```python
from build123d import *

# Parameters (mm, degrees)
BOSS_EXTRUDE3_OUTLINE_R = 7.6
BOSS_EXTRUDE3_DEPTH     = 5
SKETCH2_R               = 1.6
CUT_EXTRUDE1_DEPTH      = 10
SKETCH3_R               = 1.6
CUT_EXTRUDE2_DEPTH      = 10
SKETCH4_R               = 1.5
CUT_EXTRUDE3_DEPTH      = 10
SKETCH5_R               = 3.25
CUT_EXTRUDE4_DEPTH      = 1.5
CUT_EXTRUDE5_DEPTH      = 10
FILLET1_R               = 2
FILL_PATTERN1_DEPTH     = 5
CUT_EXTRUDE6_DEPTH      = 10
FILLET2_R               = 2
FILL_PATTERN2_DEPTH     = 5


# Read off the part's stored shape, not the designer's step: Boss-Extrude3, Fill Pattern1, Fill Pattern2
with BuildPart() as part:
    # Boss-Extrude3 outline → Boss-Extrude3 (new body)
    with BuildSketch(Plane(origin=(0, 0, 0), x_dir=(1, 0, 0), z_dir=(0, 1, 0))):
        with BuildLine():
            ThreePointArc((0, 42.5), (-42.5, 0), (0, -42.5))
            add(Edge.make_bspline(
                [(0, -42.5), (50, -42.5), (76.766110149, 8.415768242), (141.161165235, -8.838834765)],
                knots=[0, 0, 0, 0, 1, 1, 1, 1], degree=3))
            ThreePointArc((141.161165235, -8.838834765), (158.838834765, -8.838834765), (158.838834765, 8.838834765))
            add(Edge.make_bspline(
                [(0, 42.5), (53.483495706, 42.5), (123.483495706, 44.194173824), (158.838834765, 8.838834765)],
                knots=[0, 0, 0, 0, 1, 1, 1, 1], degree=3))
        make_face()
        with Locations((150, 0)):
            Circle(BOSS_EXTRUDE3_OUTLINE_R, mode=Mode.SUBTRACT)
    extrude(amount=BOSS_EXTRUDE3_DEPTH)

    # Sketch2 → Cut-Extrude1 (cut)
    with BuildSketch(Plane(origin=(0, 5, 0), x_dir=(1, 0, 0), z_dir=(0, 1, 0))):
        with Locations(Location((0, 35, 0), (0, 0, 270))):
            Circle(SKETCH2_R)
        with Locations(Location((0, 11, 0), (0, 0, 270))):
            Circle(SKETCH2_R)
        with Locations(Location((9.526279442, 5.5, 0), (0, 0, 270))):
            Circle(SKETCH2_R)
        with Locations(Location((9.526279442, -5.5, 0), (0, 0, 270))):
            Circle(SKETCH2_R)
        with Locations(Location((0, -11, 0), (0, 0, 270))):
            Circle(SKETCH2_R)
        with Locations(Location((-9.526279442, -5.5, 0), (0, 0, 270))):
            Circle(SKETCH2_R)
        with Locations(Location((-9.526279442, 5.5, 0), (0, 0, 270))):
            Circle(SKETCH2_R)
        with Locations(Location((-20.57248383, 28.315594803, 0), (0, 0, 270))):
            Circle(SKETCH2_R)
        with Locations(Location((-33.28697807, 10.815594803, 0), (0, 0, 270))):
            Circle(SKETCH2_R)
        with Locations(Location((-33.28697807, -10.815594803, 0), (0, 0, 270))):
            Circle(SKETCH2_R)
        with Locations(Location((-20.57248383, -28.315594803, 0), (0, 0, 270))):
            Circle(SKETCH2_R)
        with Locations(Location((0, -35, 0), (0, 0, 270))):
            Circle(SKETCH2_R)
    extrude(amount=-CUT_EXTRUDE1_DEPTH, mode=Mode.SUBTRACT)

    # Sketch3 → Cut-Extrude2 (cut)
    with BuildSketch(Plane(origin=(0, 5, 0), x_dir=(1, 0, 0), z_dir=(0, 1, 0))):
        with Locations(Location((29.822508304, 35, 0), (0, 0, 270))):
            Circle(SKETCH3_R)
        with Locations(Location((57.312909887, 35, 0), (0, 0, 270))):
            Circle(SKETCH3_R)
    extrude(amount=-CUT_EXTRUDE2_DEPTH, mode=Mode.SUBTRACT)

    # Sketch4 → Cut-Extrude3 (cut)
    with BuildSketch(Plane(origin=(0, 5, 0), x_dir=(1, 0, 0), z_dir=(0, 1, 0))):
        with Locations(Location((22.392043347, -28.36049342, 0), (0, 0, 270))):
            Circle(SKETCH4_R)
    extrude(amount=-CUT_EXTRUDE3_DEPTH, mode=Mode.SUBTRACT)

    # Sketch5 → Cut-Extrude4 (cut)
    with BuildSketch(Plane.XZ):
        with Locations(Location((0, 11, 0), (0, 0, 270))):
            Circle(SKETCH5_R)
        with Locations(Location((9.526279442, 5.5, 0), (0, 0, 270))):
            Circle(SKETCH5_R)
        with Locations(Location((9.526279442, -5.5, 0), (0, 0, 270))):
            Circle(SKETCH5_R)
        with Locations(Location((0, -11, 0), (0, 0, 270))):
            Circle(SKETCH5_R)
        with Locations(Location((-9.526279442, -5.5, 0), (0, 0, 270))):
            Circle(SKETCH5_R)
        with Locations(Location((-9.526279442, 5.5, 0), (0, 0, 270))):
            Circle(SKETCH5_R)
    extrude(amount=-CUT_EXTRUDE4_DEPTH, mode=Mode.SUBTRACT)

    # Sketch6 → Cut-Extrude5 (cut)
    with BuildSketch(Plane(origin=(0, 5, 0), x_dir=(1, 0, 0), z_dir=(0, 1, 0))):
        Polygon((43, 27.773502692), (23, 27.773502692), (33, 10.452994616), align=None)
    extrude(amount=-CUT_EXTRUDE5_DEPTH, mode=Mode.SUBTRACT)

    # Fillet1
    fillet1_edges = [part.edges().sort_by_distance(p)[0] for p in [
        (43, 2.5, -27.773502692),
        (33, 2.5, -10.452994616),
        (23, 2.5, -27.773502692),
    ]]
    fillet(fillet1_edges, radius=FILLET1_R)

    # Fill Pattern1 outline → Fill Pattern1 (cut)
    with BuildSketch(Plane(origin=(0, 0, 0), x_dir=(1, 0, 0), z_dir=(0, 1, 0))):
        with BuildLine():
            ThreePointArc((41.464101615, 1.792740578), (39.732050808, 0.792740578), (39.732050808, -1.207259422))
            Line((39.732050808, -1.207259422), (46.267949192, -12.527767497))
            ThreePointArc((46.267949192, -12.527767497), (48, -13.527767497), (49.732050808, -12.527767497))
            Line((49.732050808, -12.527767497), (56.267949192, -1.207259422))
            ThreePointArc((56.267949192, -1.207259422), (56.267949192, 0.792740578), (54.535898385, 1.792740578))
            Line((54.535898385, 1.792740578), (41.464101615, 1.792740578))
        make_face()
        with BuildLine():
            ThreePointArc((101.267949192, 24.773502692), (101.267949192, 26.773502692), (99.535898385, 27.773502692))
            Line((99.535898385, 27.773502692), (86.464101615, 27.773502692))
            ThreePointArc((86.464101615, 27.773502692), (84.732050808, 26.773502692), (84.732050808, 24.773502692))
            Line((84.732050808, 24.773502692), (91.267949192, 13.452994616))
            ThreePointArc((91.267949192, 13.452994616), (93, 12.452994616), (94.732050808, 13.452994616))
            Line((94.732050808, 13.452994616), (101.267949192, 24.773502692))
        make_face()
        with BuildLine():
            ThreePointArc((71.267949192, 24.773502692), (71.267949192, 26.773502692), (69.535898385, 27.773502692))
            Line((69.535898385, 27.773502692), (56.464101615, 27.773502692))
            ThreePointArc((56.464101615, 27.773502692), (54.732050808, 26.773502692), (54.732050808, 24.773502692))
            Line((54.732050808, 24.773502692), (61.267949192, 13.452994616))
            ThreePointArc((61.267949192, 13.452994616), (63, 12.452994616), (64.732050808, 13.452994616))
            Line((64.732050808, 13.452994616), (71.267949192, 24.773502692))
        make_face()
    extrude(amount=FILL_PATTERN1_DEPTH, mode=Mode.SUBTRACT)

    # Sketch8 → Cut-Extrude6 (cut)
    with BuildSketch(Plane(origin=(0, 5, 0), x_dir=(1, 0, 0), z_dir=(0, 1, 0))):
        Polygon((58, 7.56624327), (48, 24.886751346), (38, 7.56624327), align=None)
    extrude(amount=-CUT_EXTRUDE6_DEPTH, mode=Mode.SUBTRACT)

    # Fillet2
    fillet2_edges = [part.edges().sort_by_distance(p)[0] for p in [
        (58, 2.5, -7.56624327),
        (38, 2.5, -7.56624327),
        (48, 2.5, -24.886751346),
    ]]
    fillet(fillet2_edges, radius=FILLET2_R)

    # Fill Pattern2 outline → Fill Pattern2 (cut)
    with BuildSketch(Plane(origin=(0, 0, 0), x_dir=(1, 0, 0), z_dir=(0, 1, 0))):
        with BuildLine():
            ThreePointArc((69.732050808, 10.56624327), (69.732050808, 8.56624327), (71.464101615, 7.56624327))
            Line((71.464101615, 7.56624327), (84.535898385, 7.56624327))
            ThreePointArc((84.535898385, 7.56624327), (86.267949192, 8.56624327), (86.267949192, 10.56624327))
            Line((86.267949192, 10.56624327), (79.732050808, 21.886751346))
            ThreePointArc((79.732050808, 21.886751346), (78, 22.886751346), (76.267949192, 21.886751346))
            Line((76.267949192, 21.886751346), (69.732050808, 10.56624327))
        make_face()
    extrude(amount=FILL_PATTERN2_DEPTH, mode=Mode.SUBTRACT)


solid = part.part
```
The model under review builds one solid part; all positions refer to its coordinate system, in mm. A direction names the side the tool comes from. Give positions to 0.01 mm unless a question says otherwise; leave off trailing zeros. Use CSV: the item, a comma, the result in double quotes.
1. For P1, Ø6, axis at x = 9.53, z = 5.5, coming from the -Y side; P2, Ø1.5, axis at y = 3, z = -1, coming from the +X side; P3, Ø3, axis at x = 0, z = -35, coming from the +Y side; P4, Ø2, axis at y = 0.5, z = 30, coming from the -X side, all flat-tipped, find the tip position at first contact; note any pin that passes through.
Result:
P1,"stops at y = 1.5"
P2,"stops at x = 162.5"
P3,"passes through"
P4,"stops at x = -31.07"
2. The part is to be moulded in two halves that separate along X. For faces 3 (the face through (36, 0, -1)), 4 (the face through (52.954, 2.465, 6.947)), 5 (the face through (27.954, 2.535, -19.192)), say which applies: +X half, -X half, draft (parallel to the pull), parting line (faces both ways), or undercut.
Result:
face 3,"draft"
face 4,"undercut"
face 5,"undercut"
3. Machinability: for faces 1 (the face through (48, 3, -7.566)), 2 (the face through (8, 1.5, 4)), which of the approach directions +Z, -Z, +X, -X, +Y, -Y give a long, thin tool a straight path to every point of the face, cutting with its end or side? Answer none if there is none.
Result:
face 1,"+Y, -Y"
face 2,"-Y"
4. To check wall thickness, follow probe 1 along X at (y, z) = (3.15, 0); probe 2 along X at (y, z) = (0.7, -11); probe 3 along Z at (x, y) = (85, 3.4). State the ranges of each line that lie inside material, in increasing order. Write a range as from..to.
Result:
probe 1,"x = -42.5..39.47, 56.53..142.4, 157.6..162.5"
probe 2,"x = -41.05..-34.88, -31.7..-3.25, 3.25..39.98, 56.02..69.98, 86.02..156.59"
probe 3,"z = -39.09..-27.14, -24.31..-12.76, -7.62..10.59"
5. Consider section A-A, the plane y = 3.45. Count the separate pieces of the cut face and the enclosed holes in it, then the cut area to 3 significant figures.
Result:
separate pieces,"1"
enclosed holes,"22"
area,"10,300 mm²"
